For this review, use the dimensioned drawing (mm, ordinates from the lowest corner) and the shaded views. A direction names the side the tool comes from. Give positions to 0.01 mm unless a question says otherwise; leave off trailing zeros. Write each loop counter-clockwise with the first axis right and the second up, starting at its lowest first coordinate (ties: lowest second). Pieces come first, ordered by that corner, then holes. Notation, with made-up numbers: M -11,55.5 L 46,55.5 A32 cw 46,87.5 Z; hole C -37.75,-23.75 d6. An arc over 180 degrees is marked long. One line per item, written item: value. Start each with the question number.
Item 1: Mouldability with a two-part tool opening along Z and no side actions: class the marked faces 4, 5 and 6 as released by +Z, released by -Z, zero draft, split by the parting line, or undercut.
Item 2: Tool access review of the marked faces 1, 2 and 3: name each direction out of +Z, -Z, +X, -X, +Y, -Y from which nothing blocks a thin tool from reaching the whole face with its end or side.
Item 3: To check wall thickness, follow probe 1 along Y at (x, z) = (6.5, 1.5); probe 2 along Z at (x, y) = (5.75, 1.05); probe 3 along Z at (x, y) = (5.5, 3.5). State the ranges of each line that lie inside material, in increasing order.
Item 4: Consider section C-C, the plane y = 0.8. Write out the cut boundary in (x, z).
Item 5: Consider section D-D, the plane y = 4.25. Write out the cut boundary in (x, z), and give its area (3 significant figures).
Item 6: Consider section B-B, the plane z = 5. Write out the cut boundary in (x, y).
Item 7: Consider section A-A, the plane x = 5. Write out the cut boundary in (y, z), and give its area (3 significant figures).
Item 8: Clearance check with flat-ended pins moving along their axes: pin 1 Ø1.5 at (x, y) = (3, 3) entering from -Z; pin 2 Ø0.7 at (y, z) = (2, 3) entering from +X; pin 3 Ø2 at (y, z) = (3, 3) entering from +X. State where each tip first meets the part, or that it passes through.
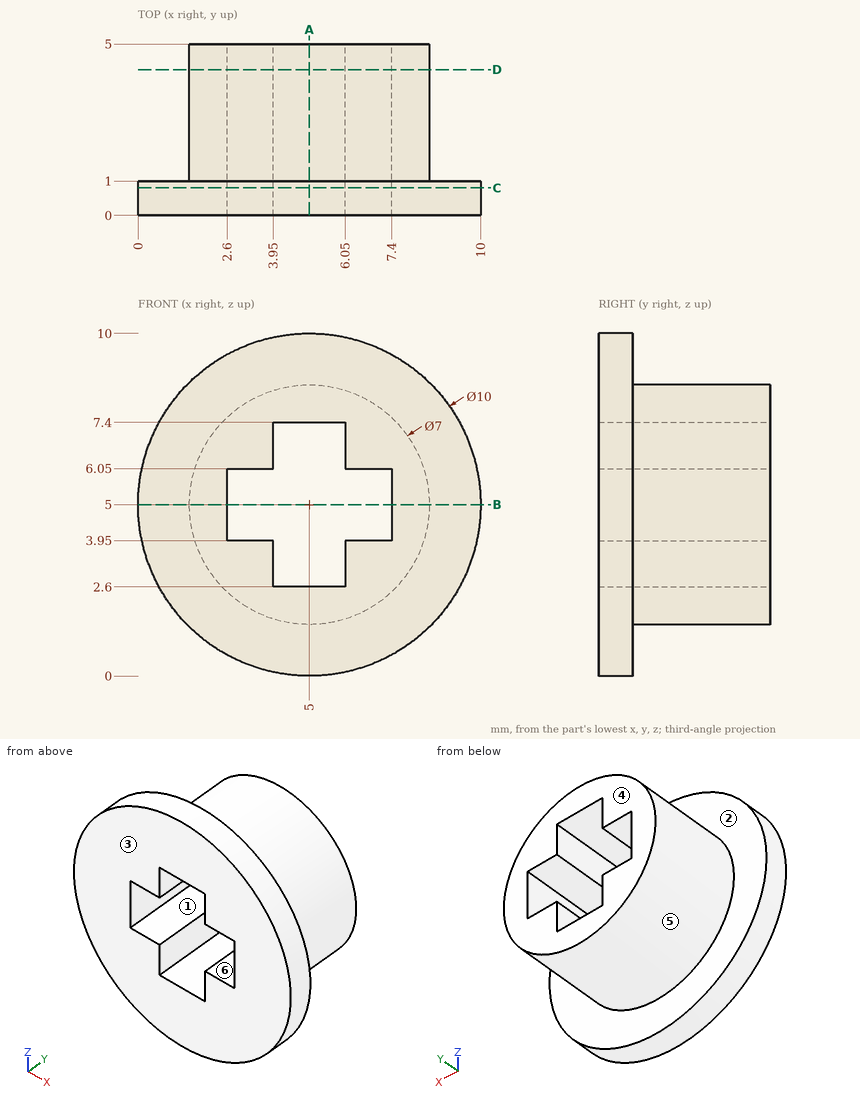
Model answer:
1. face 4: zero draft
1. face 5: split by the parting line
1. face 6: undercut
2. face 1: +Y, -Y
2. face 2: +Y
2. face 3: +Z, -Z, +X, -X, -Y
3. probe 1: y = 0 to 1
3. probe 2: z = 1.58 to 2.6, 7.4 to 8.42
3. probe 3: z = 1.54 to 2.6, 7.4 to 8.46
4. outline: C 5,5 d10; hole M 2.6,3.95 L 3.95,3.95 L 3.95,2.6 L 6.05,2.6 L 6.05,3.95 L 7.4,3.95 L 7.4,6.05 L 6.05,6.05 L 6.05,7.4 L 3.95,7.4 L 3.95,6.05 L 2.6,6.05 Z
5. outline: C 5,5 d7; hole M 2.6,3.95 L 3.95,3.95 L 3.95,2.6 L 6.05,2.6 L 6.05,3.95 L 7.4,3.95 L 7.4,6.05 L 6.05,6.05 L 6.05,7.4 L 3.95,7.4 L 3.95,6.05 L 2.6,6.05 Z
5. area: 22.7 mm2
6. outline: M 0,0 L 2.6,0 L 2.6,5 L 1.5,5 L 1.5,1 L 0,1 Z; M 7.4,0 L 10,0 L 10,1 L 8.5,1 L 8.5,5 L 7.4,5 Z
7. outline: M 0,0 L 1,0 L 1,1.5 L 5,1.5 L 5,2.6 L 0,2.6 Z; M 0,7.4 L 5,7.4 L 5,8.5 L 1,8.5 L 1,10 L 0,10 Z
7. area: 14.0 mm2
8. pin 1: stops at z = 1.73
8. pin 2: stops at x = 8.09
8. pin 3: stops at x = 8.35
